Input: part model. Units: mm. Frame: model coordinates. A direction names the side the tool comes from. Round coordinates to 2 decimals unless told otherwise and drop trailing zeros. Loops run counter-clockwise (first coordinate to the right, second up) from the corner with the lowest first, then second, coordinate; pieces in that order, holes last. Notation, with made-up numbers: (13, 53) -> (39, 53) arc R20 ccw to (39, 91) -> close; hole circle Ø5 at (44.5, 28.25). An arc over 180 degrees is marked (long way). Answer as a JSON object with one key per item and string values. Group by question number.
Item 1: Draft query along Z for faces 1 (the flat face through (-4, 1.651, 0)), 2 (the cylindrical face through (1.572, 1.803, 0.652)), 3 (the flat face through (0, 2, -16.51)). Return one class per face: released by +Z, released by -Z, zero draft, split by the parting line, or undercut.
Item 2: Section query A-A on z = 0. Return loops of the section in (x, y), and give its area (3 significant figures).
Item 3: Section query C-C on y = 0.65. Return loops of the section in (x, z).
Item 4: Set-up query: faces 4 (the flat face through (4, 1.651, 0)), 5 (the flat face through (2, 3.556, 0)), 6 (the flat face through (-2.997, 3, 0)). Return all of +Z, -Z, +X, -X, +Y, -Y with unobstructed straight access to the full face (end or side cutting, diameter ignored); none if empty.
Item 5: Material intervals for line 1 (Z direction, x = 0, y = 1.75); line 2 (Z direction, x = 1.25, y = 0.95); line 3 (X direction, y = 2.8, z = -8), sorted ascending. Write a range as [from, to].
Item 6: Pin query (flat end, axial travel): pin 1 (1.5 mm diameter, centred on y = 2.5, z = -7.5, fed in from +X); pin 2 (1 mm diameter, centred on y = 3, z = 7, fed in from -X); pin 3 (1.1 mm diameter, centred on x = -4, z = -8, fed in from +Y). Return the tip coordinate at first contact, or that it passes through.
Item 7: Section query B-B on x = 0. Return loops of the section in (y, z).
Item 8: Section query D-D on z = 6. Return loops of the section in (x, y), and give its area (3 significant figures).
Autodesk Inventor part; units mm, degrees
ref_plane "XZ Plane" through (0, 0, 0) normal (0, 1, 0) x (-1, 0, 0)
ref_plane "XY Plane" through (0, 0, 0) normal (0, 0, 1) x (1, 0, 0)
sketch "Sketch1" plane through (0, 0, 0) normal (0, 1, 0) x (-1, 0, 0)
  line L0 (4.318, 16.51) -> (-4.318, 16.51)
  line L1 (-4.318, 16.51) -> (-4.318, -16.51)
  line L2 (-4.318, -16.51) -> (4.318, -16.51)
  line L3 (4.318, -16.51) -> (4.318, 16.51)
  line L4 (4.318, 16.51) -> (-4.318, -16.51) construction
  line L5 (-4.318, 16.51) -> (4.318, -16.51) construction
  point P0 (0, 0)
  dimension "d0" = 8.636
  dimension "d1" = 33.02
extrude "Base" add sketch "Sketch1" along normal blind 1.651
sketch "Sketch2" plane through (0, 1.651, 0) normal (0, 1, 0) x (1, 0, 0)
  line L0 (-2.9972, -16.51) -> (2.9972, -16.51)
  line L1 (2.9972, -16.51) -> (2.9972, 16.51)
  line L2 (2.9972, 16.51) -> (-2.9972, 16.51)
  line L3 (-2.9972, 16.51) -> (-2.9972, -16.51)
  line L4 (-2.9972, -16.51) -> (2.9972, 16.51) construction
  line L5 (2.9972, -16.51) -> (-2.9972, 16.51) construction
  point P0 (0, 0)
  dimension "d4" = 5.9944
  dimension "d5" = 33.02
extrude "Step" add sketch "Sketch2" along normal blind 1.905
sketch "Sketch3" plane through (0, 3.556, 0) normal (0, 1, 0) x (1, 0, 0)
  circle A0 centre (0, 0) radius 1.7018
  circle A1 centre (0, -9.779) radius 1.7018
  circle A2 centre (0, 9.779) radius 1.7018
  dimension "d8" = 3.4036
  dimension "d9" = 3.4036
  dimension "d10" = 3.4036
  dimension "d11" = 9.779
  dimension "d12" = 9.779
extrude "Holes" cut sketch "Sketch3" against normal through all
properties part number "585757_plastic_770_holes"
Solved:
{
 "1": {"face 1": "zero draft", "face 2": "undercut", "face 3": "released by -Z"},
 "2": {"outline": "(-4.32, 0) -> (-1.7, 0) -> (-1.7, 3.56) -> (-3, 3.56) -> (-3, 1.65) -> (-4.32, 1.65) -> close; (1.7, 0) -> (4.32, 0) -> (4.32, 1.65) -> (3, 1.65) -> (3, 3.56) -> (1.7, 3.56) -> close", "area": "13.6 mm²"},
 "3": {"outline": "(-4.32, -16.51) -> (4.32, -16.51) -> (4.32, 16.51) -> (-4.32, 16.51) -> close; hole circle Ø3.4 at (0, -9.78); hole circle Ø3.4 at (0, 0); hole circle Ø3.4 at (0, 9.78)"},
 "4": {"face 4": "+Z, -Z, +X, +Y", "face 5": "+Z, -Z, +X, -X, +Y", "face 6": "+Z, -Z, -X, +Y"},
 "5": {"line 1": "[-16.51, -11.48], [-8.08, -1.7], [1.7, 8.08], [11.48, 16.51]", "line 2": "[-16.51, -10.93], [-8.62, -1.15], [1.15, 8.62], [10.93, 16.51]", "line 3": "[-3, 3]"},
 "6": {"pin 1": "x = 3", "pin 2": "x = -3", "pin 3": "y = 1.65"},
 "7": {"outline": "(0, -16.51) -> (3.56, -16.51) -> (3.56, -11.48) -> (0, -11.48) -> close; (0, -8.08) -> (3.56, -8.08) -> (3.56, -1.7) -> (0, -1.7) -> close; (0, 1.7) -> (3.56, 1.7) -> (3.56, 8.08) -> (0, 8.08) -> close; (0, 11.48) -> (3.56, 11.48) -> (3.56, 16.51) -> (0, 16.51) -> close"},
 "8": {"outline": "(-4.32, 0) -> (4.32, 0) -> (4.32, 1.65) -> (3, 1.65) -> (3, 3.56) -> (-3, 3.56) -> (-3, 1.65) -> (-4.32, 1.65) -> close", "area": "25.7 mm²"}
}
